from build123d import *

# Parameters (mm, degrees)
F0_R     = 25
F1_DEPTH = 101.516215
F2_R     = 12.537375
F3_DEPTH = 50.175298
F4_R     = 17.345537
F5_DEPTH = 56.003423


with BuildPart() as f1:
    # F0 (on Front) → F1 (new body)
    with BuildSketch(Plane.XZ):
        Circle(F0_R)
    extrude(amount=F1_DEPTH)

    # F2 (on face) → F3 (cut)
    with BuildSketch(Plane(origin=(0, 0, 0), x_dir=(-1, 0, 0), z_dir=(0, 1, 0))):
        Circle(F2_R)
    extrude(amount=-F3_DEPTH, mode=Mode.SUBTRACT)

    # F4 (on face) → F5 (cut)
    with BuildSketch(Plane.XZ.offset(101.516215)):
        Circle(F4_R)
    extrude(amount=-F5_DEPTH, mode=Mode.SUBTRACT)


solid = f1.part
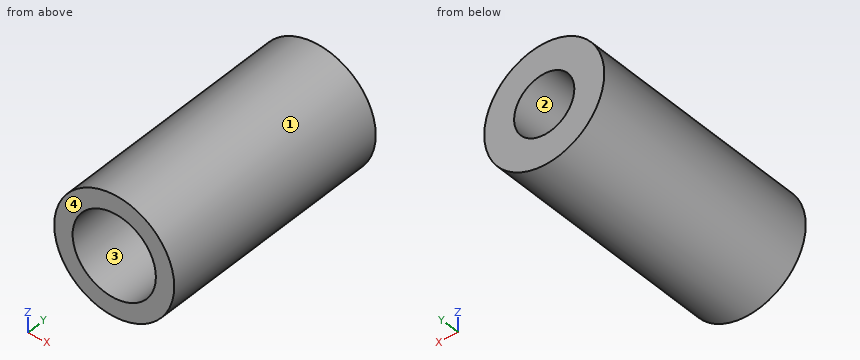
The model under review builds one solid part; all positions refer to its coordinate system, in mm. Face numbers are marked on the shaded views. Give positions to 0.01 mm unless a question says otherwise; leave off trailing zeros. Write each loop counter-clockwise with the first axis right and the second up, starting at its lowest first coordinate (ties: lowest second). Pieces come first, ordered by that corner, then holes.
1. For P1, Ø20, axis at x = 0, z = 0, coming from the -Y side; P2, Ø8, axis at x = -19, y = -36.5, coming from the -Z side; P3, Ø1.5, axis at y = -42.5, z = -15, coming from the +X side; P4, Ø3, axis at x = 5.5, y = -78, coming from the +Z side, all flat-tipped, find the tip position at first contact; note any pin that passes through.
2. Draft analysis for pull direction X (two halves, no side actions). For the marked faces 1, 2, 3 and 4, state which applies: +X half, -X half, draft (parallel to the pull), parting line (faces both ways), or undercut.
3. Add section B-B, the plane x = 0. Write out the cut boundary in (y, z).
4. Add section A-A, the plane z = 0. Write out the cut boundary in (x, y).
5. Add section D-D, the plane z = 14.5. Write out the cut boundary in (x, y).
6. Wall thickness on L1, parallel to Z at x = 0, y = -69; L2, parallel to Z at x = 0, y = -31; L3, parallel to Y at x = -7, z = -15: over which ranges is each line inside the solid? List them lowest first.
7. Add section C-C, the plane y = -25. Write out the cut boundary in (x, z), plus the area to 3 significant figures.
Worked answers:
1. P1: passes through
1. P2: stops at z = -20
1. P3: stops at x = 20.54
1. P4: stops at z = 24.68
2. face 1: parting line
2. face 2: undercut
2. face 3: undercut
2. face 4: draft
3. outline: (-101.52, -25) - (0, -25) - (0, -12.54) - (-45.51, -12.54) - (-45.51, -17.35) - (-101.52, -17.35) - close; (-101.52, 17.35) - (-45.51, 17.35) - (-45.51, 12.54) - (0, 12.54) - (0, 25) - (-101.52, 25) - close
4. outline: (-25, -101.52) - (-17.35, -101.52) - (-17.35, -45.51) - (-12.54, -45.51) - (-12.54, 0) - (-25, 0) - close; (12.54, -45.51) - (17.35, -45.51) - (17.35, -101.52) - (25, -101.52) - (25, 0) - (12.54, 0) - close
5. outline: (-20.37, -101.52) - (-9.52, -101.52) - (-9.52, -45.51) - (9.52, -45.51) - (9.52, -101.52) - (20.37, -101.52) - (20.37, 0) - (-20.37, 0) - close
6. L1: z = -25 to -17.35, 17.35 to 25
6. L2: z = -25 to -12.54, 12.54 to 25
6. L3: y = -45.51 to 0
7. outline: circle Ø50 at (0, 0); hole circle Ø25.07 at (0, 0)
7. area: 1,470 mm2
